The listing builds one solid part. Answer for the finished solid, in the listing's coordinates (mm). A direction names the side the tool comes from. Round coordinates to 2 decimals unless told otherwise and drop trailing zeros. Loops run counter-clockwise (first coordinate to the right, second up) from the corner with the lowest first, then second, coordinate; pieces in that order, holes last. Notation, with made-up numbers: (31.25, -33) -> (56.25, -33) arc R15 cw to (56.25, -13) -> close; hole circle Ø3 at (66.25, -21.5). An arc over 180 degrees is marked (long way). Use a Markdown table: item, result. Add a question column.
Q1. Section A-A on x = 53.5 is taken. Give the vertices of the cut face in (y, z), then the cut area to 3 significant figures.
Q2. Section C-C on x = -8 is taken. Give the vertices of the cut face in (y, z), then the cut area to 3 significant figures.
Q3. Consider line 1 (Z direction, x = -41.5, y = -25.5); line 2 (X direction, y = -31.5, z = -40); line 3 (X direction, y = -81, z = 51). Determine where each line is inside the solid, lowest interval first.
Q4. Section B-B on y = -49 is taken. Give the number of separate pieces and of enclosed holes in the cut face, then the cut area to 3 significant figures.
Q5. Section D-D on z = -51 is taken. Give the vertices of the cut face in (x, y), then the cut area to 3 significant figures.
Q6. Given pin 1 Ø19 at (y, z) = (-74.5, 31.5) entering from +X; pin 2 Ø4 at (x, y) = (42, -109.5) entering from +Z; pin 3 Ø5 at (x, y) = (22.5, -17.5) entering from +Z, each flat-ended and moving along its own axis, determine where each tip first touches the part or whether it passes through.
Q7. Which of the six approach directions +Z, -Z, +X, -X, +Y, -Y give full straight-line access (tool end or side, diameter ignored) to faces 1 (the flat face through (-51.232, -62.611, 67.696)), 2 (the flat face through (-2, -127, 42))?
Q8. For a pull along Z with two mould halves and no side action, classify faces 3 (the flat face through (-39, -63, -75.753)), 4 (the flat face through (31, -63, 56.099)), 5 (the flat face through (-2, 0, 42)) as released by +Z, released by -Z, zero draft, split by the parting line, or undercut.
from build123d import *

# Parameters (mm, degrees)
F0_W     = 38.259773
F0_H     = 38.259772
F0_W_2   = 38.259772
F1_DEPTH = 127


with BuildPart() as f1:
    # F0 (on Front) → F1 (new body)
    with BuildSketch(Plane.XZ):
        Polygon((-1.480275, -75.753056), (-63.029461, -18.419569), (0, -67.634352), (63.677665, -19.261191), (1.517248, -75.753056), (75.698244, -75.753056), (75.698244, 76.035975), (-76.445349, 76.268949), (-76.445349, -75.753056), align=None)
        with Locations((-37.750917, 36.969415)):
            Rectangle(F0_W, F0_H, mode=Mode.SUBTRACT)
        with Locations((31.434221, 36.969415)):
            Rectangle(F0_W_2, F0_H, mode=Mode.SUBTRACT)
        Polygon((-49.296099, 65.077743), (-53.221939, 70.389176), (-50.653815, 73.10266), (-47.200143, 70.389176), (-44.124323, 74.304022), (-41.230742, 70.389176), (-36.907537, 73.584587), (-31.946439, 70.389176), (-26.044864, 74.751208), (-25.51012, 66.232399), (-30.821553, 62.306558), (-34.747393, 67.617991), (-40.058826, 63.692151), (-43.984666, 69.003583), align=None, mode=Mode.SUBTRACT)
        Polygon((23.569294, 64.333276), (18.898987, 69.003583), (18.898987, 73.10266), (21.928739, 69.003583), (28.239602, 75.314446), (34.550464, 69.003583), (38.649541, 73.10266), (42.748618, 69.003583), (46.847696, 73.10266), (46.92083, 69.003583), (42.250523, 64.333276), (37.580216, 69.003583), (32.909909, 64.333276), (28.239602, 69.003583), align=None, mode=Mode.SUBTRACT)
        Polygon((-46.067663, 132.356301), (-76.445349, 76.268949), (75.698244, 76.035975), (46.18622, 132.583613), (0, 156.528115), align=None)
        Polygon((0, 156.528115), (46.18622, 132.583613), (85.278795, 152.985897), align=None)
        Polygon((85.278795, 152.985897), (46.18622, 132.583613), (97.734198, 111.462012), align=None)
        Polygon((108.309702, 120.26045), (85.278795, 152.985897), (97.734198, 111.462012), (108.591035, 119.860694), align=None)
        with BuildLine():
            Line((108.591035, 119.860694), (97.734198, 111.462012))
            ThreePointArc((97.734198, 111.462012), (115.323637, 101.074909), (108.309702, 120.26045))
            Line((108.309702, 120.26045), (108.591035, 119.860694))
        make_face()
    extrude(amount=F1_DEPTH)


solid = f1.part
Checked values:
| question | item | result |
|---|---|---|
| 1 | outline | (-127, -75.75) -> (0, -75.75) -> (0, -28.51) -> (-127, -28.51) -> close; (-127, -26.99) -> (0, -26.99) -> (0, 118.57) -> (-127, 118.57) -> close; (-127, 129.59) -> (0, 129.59) -> (0, 154.31) -> (-127, 154.31) -> close |
| 1 | area | 27,600 mm2 |
| 2 | outline | (-127, -75.75) -> (0, -75.75) -> (0, -69.68) -> (-127, -69.68) -> close; (-127, -61.39) -> (0, -61.39) -> (0, 152.33) -> (-127, 152.33) -> close |
| 2 | area | 27,900 mm2 |
| 3 | line 1 | z = -75.75 to -38.47, -35.23 to 17.84, 56.1 to 65.64, 70.75 to 134.75 |
| 3 | line 2 | x = -76.45 to -39.86, -35.39 to 36.38, 40.86 to 75.7 |
| 3 | line 3 | x = -76.45 to -56.88, -18.62 to 12.3, 50.56 to 75.7 |
| 4 | separate pieces | 1 |
| 4 | enclosed holes | 4 |
| 4 | area | 29,800 mm2 |
| 5 | outline | (-76.45, -127) -> (-28.05, -127) -> (-28.05, 0) -> (-76.45, 0) -> close; (-21.3, -127) -> (21.9, -127) -> (21.9, 0) -> (-21.3, 0) -> close; (28.75, -127) -> (75.7, -127) -> (75.7, 0) -> (28.75, 0) -> close |
| 5 | area | 17,600 mm2 |
| 6 | pin 1 | stops at x = 75.7 |
| 6 | pin 2 | stops at z = 154.87 |
| 6 | pin 3 | stops at z = 155.7 |
| 7 | face 1 | +Y, -Y |
| 7 | face 2 | +Z, -Z, +X, -X, -Y |
| 8 | face 3 | released by -Z |
| 8 | face 4 | undercut |
| 8 | face 5 | zero draft |
